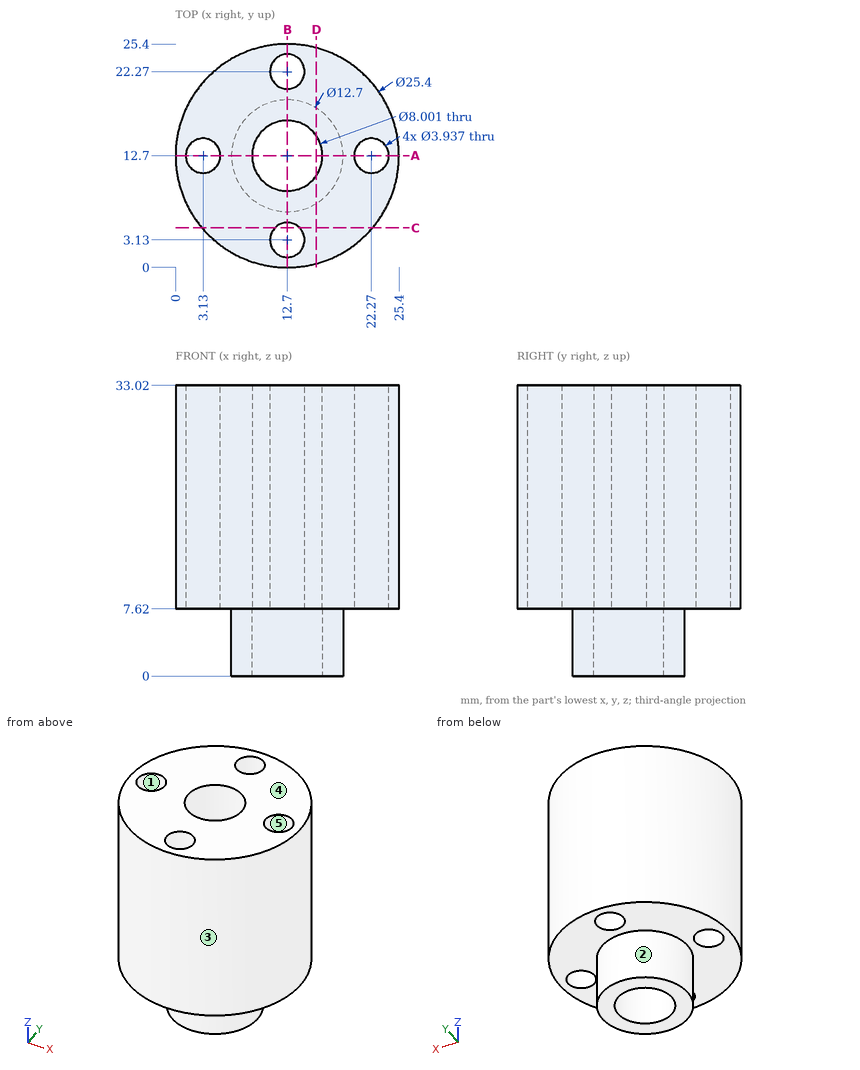
Geometry: see drawing. Coordinates: mm, zero at the bounding-box minimum. A direction names the side the tool comes from. Give positions to 0.01 mm unless a question says otherwise; leave off trailing zeros. Order: outer loops, then holes, each group sorted by start corner. A loop starts at its lowest first (then second) coordinate and runs counter-clockwise, first axis right, second up. Notation, with made-up numbers: M 18.5,11 L 70.5,11 A19 ccw 70.5,41 Z; hole C -31,-34 d4. An arc over 180 degrees is marked long. Answer as CSV lines item,"result". Start each with the question number.
1) Set-up query: the marked faces 1 and 2. Return all of +Z, -Z, +X, -X, +Y, -Y with unobstructed straight access to the full face (end or side cutting, diameter ignored); none if empty.
2) First-contact query: P1, Ø2, axis at x = 10.5, z = 26, coming from the +Y side; P2, Ø6, axis at y = 4, z = 6.5, coming from the +X side; P3, Ø2.5, axis at x = 12.7, y = 22.27, coming from the +Z side; P4, Ø2, axis at y = 3.5, z = 13.5, coming from the -X side. Flat tips, straight axial feed; report the tip coordinate or a pass-through.
3) Mould query, pull axis X, two halves, no side actions, for the marked faces 3, 4 and 5. Classes: +X half, -X half, draft (parallel to the pull), parting line (faces both ways), or undercut.
4) Line query: line 1 (Y direction, x = 12.7, z = 26); line 2 (Y direction, x = 15, z = 23); line 3 (Z direction, x = 2.5, y = 16.5). Output: solid intervals per line, ascending. Write a range as from..to.
5) Cut plane D-D (x = 16). Output: boundary loops of the cut face in (y, z) (1 decimal).
6) Cut plane A-A (y = 12.7). Output: boundary loops of the cut face in (x, z), then the cut area to 3 significant figures.
7) Cut plane C-C (y = 4.5). Output: boundary loops of the cut face in (x, z), then the cut area to 3 significant figures.
Findings below:
1,face 1,"+Z, -Z"
1,face 2,"-Z"
2,P1,"stops at y = 25.34"
2,P2,"stops at x = 23.94"
2,P3,"passes through"
2,P4,"stops at x = 3"
3,face 3,"parting line"
3,face 4,"draft"
3,face 5,"undercut"
4,line 1,"y = 0..1.16, 5.1..8.7, 16.7..20.3, 24.24..25.4"
4,line 2,"y = 0.21..9.43, 15.97..25.19"
4,line 3,"z = 7.62..33.02"
5,outline,"M 0.4,7.6 L 7.3,7.6 L 7.3,0 L 10.4,0 L 10.4,33 L 0.4,33 Z; M 15,0 L 18.1,0 L 18.1,7.6 L 25,7.6 L 25,33 L 15,33 Z"
6,outline,"M 0,7.62 L 1.16,7.62 L 1.16,33.02 L 0,33.02 Z; M 5.1,7.62 L 6.35,7.62 L 6.35,0 L 8.7,0 L 8.7,33.02 L 5.1,33.02 Z; M 16.7,0 L 19.05,0 L 19.05,7.62 L 20.3,7.62 L 20.3,33.02 L 16.7,33.02 Z; M 24.24,7.62 L 25.4,7.62 L 25.4,33.02 L 24.24,33.02 Z"
6,area,"278 mm²"
7,outline,"M 3,7.62 L 11.29,7.62 L 11.29,33.02 L 3,33.02 Z; M 14.11,7.62 L 22.4,7.62 L 22.4,33.02 L 14.11,33.02 Z"
7,area,"421 mm²"
